```python
from build123d import *

# Parameters (mm, degrees)
EXTRUDE_THIN1_DEPTH = 23.5
BOSS_EXTRUDE1_DEPTH = 7


with BuildPart() as part:
    # Sketch2 → Extrude-Thin1 (new, symmetric)
    with BuildSketch(Plane.XY):
        with BuildLine():
            Line((17.163468236, -58.085931667), (-17.281893756, -13.288195823))
            ThreePointArc((-17.281893756, -13.288195823), (-19.897637951, 8.906402414), (-1.60242719, 21.741026358))
            Line((-1.60242719, 21.741026358), (117.263507159, 30.502066523))
            ThreePointArc((117.263507159, 30.502066523), (118.105083127, 30.537349971), (118.94720479, 30.519290718))
            Line((118.94720479, 30.519290718), (229.299625502, 24.652631518))
            ThreePointArc((229.299625502, 24.652631518), (244.976573908, 13.975728829), (242.768549107, -4.862731534))
            Line((242.768549107, -4.862731534), (200.935093877, -58.602091631))
            ThreePointArc((200.935093877, -58.602091631), (194.508519277, -63.812915391), (186.443863356, -65.660852138))
            Line((186.443863356, -65.660852138), (31.619949002, -65.231091278))
            ThreePointArc((31.619949002, -65.231091278), (23.562249738, -63.336718399), (17.163468236, -58.085931667))
        make_face()
        with BuildLine():
            Line((17.71839143, -57.65924648), (-16.726970562, -12.861510636))
            ThreePointArc((-16.726970562, -12.861510636), (-19.258722971, 8.620417015), (-1.550973106, 21.042920007))
            Line((-1.550973106, 21.042920007), (117.314961243, 29.803960172))
            ThreePointArc((117.314961243, 29.803960172), (118.112243739, 29.837386596), (118.910043209, 29.820277831))
            Line((118.910043209, 29.820277831), (229.262463921, 23.95361863))
            ThreePointArc((229.262463921, 23.95361863), (244.339747634, 13.685122055), (242.216182798, -4.432741463))
            Line((242.216182798, -4.432741463), (200.382727568, -58.17210156))
            ThreePointArc((200.382727568, -58.17210156), (194.201978227, -63.183604192), (186.445806412, -64.960854834))
            Line((186.445806412, -64.960854834), (31.621892057, -64.531093975))
            ThreePointArc((31.621892057, -64.531093975), (23.872410798, -62.709183447), (17.71839143, -57.65924648))
        make_face(mode=Mode.SUBTRACT)
    extrude(amount=EXTRUDE_THIN1_DEPTH, both=True)

    # Sketch3 → Boss-Extrude1 (add)
    with BuildSketch(Plane.XY.offset(23.5)):
        with BuildLine():
            Line((-15.342607214, -3.774175921), (-14.921356346, 5.195490812))
            Line((-14.921356346, 5.195490812), (-18.814600986, 9.982348011))
            Line((-18.814600986, 9.982348011), (-19.366834284, 10.008283061))
            ThreePointArc((-19.366834284, 10.008283061), (-21.78121341, 0.904843849), (-20.130207607, -8.367481205))
            Line((-20.130207607, -8.367481205), (-19.667345501, -8.175084284))
            Line((-19.667345501, -8.175084284), (-15.342607214, -3.774175921))
        make_face()
    extrude(amount=-BOSS_EXTRUDE1_DEPTH)


solid = part.part
```
The listing builds one solid part. Answer for the finished solid, in the listing's coordinates (mm). A direction names the side the tool comes from. Give positions to 0.01 mm unless a question says otherwise; leave off trailing zeros. Loops run counter-clockwise (first coordinate to the right, second up) from the corner with the lowest first, then second, coordinate; pieces in that order, holes last. Notation, with made-up numbers: (-23.5, -5.5) - (-5.5, -5.5) arc R18 ccw to (-5.5, 19.5) - close; hole circle Ø2 at (30, 89.25). An arc over 180 degrees is marked (long way). Return JSON: item names as keys, results as strings. Group by question number.
1. Find section B-B (y = -53). Write down the section's boundary in (x, z).
2. Determine the mould class of faces 4 (the cylindrical face through (244.226, 13.929, 0.329)), 5 (the flat face through (0.18, -36, 0.33)), 6 (the flat face through (222.14, -31.36, 0.33)), 7 (the flat face through (52.1, 25.4, 23.5)) for opening direction X: pulls with the +X half, pulls with the -X half, needs draft (parallel to the pull), parting line crosses it, or undercut.
3. Which of the six approach directions +Z, -Z, +X, -X, +Y, -Y give full straight-line access (tool end or side, diameter ignored) to faces 1 (the cylindrical face through (-19.4, 8.3, 0.3)), 2 (the cylindrical face through (194.303, -63.134, 0.329)), 3 (the flat face through (57, 26.06, 0.33))?
4. Find section A-A (z = 7.5). Write down the section's boundary in (x, y), then the cut area to 3 significant figures.
5. Find section C-C (x = 107). Write down the section's boundary in (y, z), then the cut area to 3 significant figures.
6. Straight lines are drawn through the part: line 1 (Y direction, x = 82.5, z = -17.5); line 2 (X direction, y = -15, z = -2.5); line 3 (Y direction, x = 197.5, z = -20). For each, find the intervals that lie inside material, in ascending order. Write a range as [from, to].
7. Given pin 1 Ø1 at (x, z) = (179, 11.5) entering from -Y; pin 2 Ø10 at (x, z) = (67, -14.5) entering from -Y; pin 3 Ø6 at (x, y) = (18, 16.5) entering from -Z; pin 4 Ø10 at (y, z) = (-7, 17) entering from +X, each flat-ended and moving along its own axis, determine where each tip first touches the part or whether it passes through.
Verdict:
{
 "1": {"outline": "(13.25, -23.5) - (14.14, -23.5) - (14.14, 23.5) - (13.25, 23.5) - close; (204.41, -23.5) - (205.3, -23.5) - (205.3, 23.5) - (204.41, 23.5) - close"},
 "2": {"face 4": "undercut", "face 5": "pulls with the -X half", "face 6": "pulls with the +X half", "face 7": "needs draft"},
 "3": {"face 1": "-Z", "face 2": "+Z, -Z", "face 3": "+Z, -Z, -X, +Y"},
 "4": {"outline": "(-17.28, -13.29) - (17.16, -58.09) arc R18.3 ccw to (31.62, -65.23) - (186.44, -65.66) arc R18.3 ccw to (200.94, -58.6) - (242.77, -4.86) arc R18.3 ccw to (229.3, 24.65) - (118.95, 30.52) arc R13.3 ccw to (117.26, 30.5) - (-1.6, 21.74) arc R21.8 ccw to start; hole (-16.73, -12.86) - (17.72, -57.66) arc R17.6 ccw to (31.62, -64.53) - (186.45, -64.96) arc R17.6 ccw to (200.38, -58.17) - (242.22, -4.43) arc R17.6 ccw to (229.26, 23.95) - (118.91, 29.82) arc R12.6 ccw to (117.31, 29.8) - (-1.55, 21.04) arc R21.1 ccw to start", "area": "440 mm^2"},
 "5": {"outline": "(-65.44, -23.5) - (-64.74, -23.5) - (-64.74, 23.5) - (-65.44, 23.5) - close; (29.04, -23.5) - (29.75, -23.5) - (29.75, 23.5) - (29.04, 23.5) - close", "area": "65.9 mm^2"},
 "6": {"line 1": "y = [-65.37, -64.67], [27.24, 27.94]", "line 2": "x = [-15.97, -15.08], [233.99, 234.88]", "line 3": "y = [-61.98, -61.1], [25.64, 26.34]"},
 "7": {"pin 1": "stops at y = -65.64", "pin 2": "stops at y = -65.34", "pin 3": "passes through", "pin 4": "stops at x = 244.6"}
}
